Geometry: see drawing. Coordinates: mm, zero at the bounding-box minimum. Give positions to 0.01 mm unless a question says otherwise; leave off trailing zeros. Loops run counter-clockwise (first coordinate to the right, second up) from the corner with the lowest first, then second, coordinate; pieces in that order, holes last. Notation, with made-up numbers: (50.5, 48) - (82.5, 48) arc R13 ccw to (82.5, 70) - close; hole circle Ø3 at (70, 71.25). An arc over 180 degrees is marked (long way). Use one line per item in the form item = value.
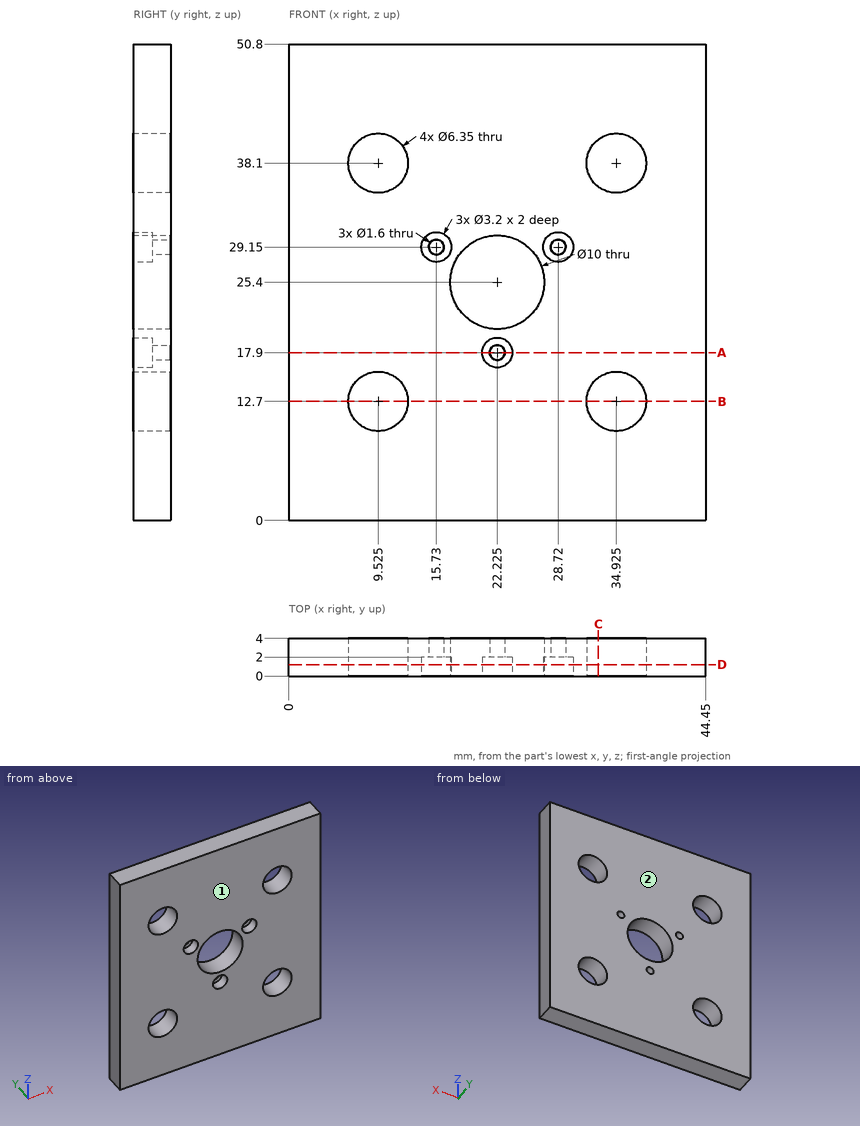
(1) Cut plane A-A (z = 17.9). Return the cut outline in (x, y) (3 decimals), plus the area to 3 significant figures.
Solution:
outline = (0, 0) - (20.625, 0) - (20.625, 2) - (21.425, 2) - (21.425, 4) - (0, 4) - close; (23.025, 2) - (23.825, 2) - (23.825, 0) - (44.45, 0) - (44.45, 4) - (23.025, 4) - close
area = 168 mm2
(2) Pull-direction query (Y, two-part tool) for the marked faces 1 and 2; classes: released by +Y, released by -Y, zero draft, split by the parting line, or undercut.
Solution:
face_1 = released by -Y
face_2 = released by +Y
(3) Material intervals for L1, parallel to X at y = 1.6, z = 38; L2, parallel to X at y = 0.85, z = 17.9 (3 decimals); L3, parallel to Z at x = 7.5, y = 3.1 (1 decimal), sorted ascending. Write a range as from..to.
Solution:
L1 = 0..6.35, 12.7..31.75, 38.1..44.45
L2 = 0..20.625, 23.825..44.45
L3 = 0..10.3, 15.1..35.7, 40.5..50.8
(4) Pin query (flat end, axial travel): P1, Ø1, axis at x = 28.5, z = 30, coming from the -Y side. Return the tip coordinate at first contact, or that it passes through.
Solution:
P1 = 2
(5) Cut plane D-D (y = 1.2). Give the number of separate pieces and of enclosed holes in the cut face, plus the area to 3 significant figures.
Solution:
separate_pieces = 1
enclosed_holes = 8
area = 2,030 mm2
(6) Cut plane B-B (z = 12.7). Return the cut outline in (x, y), plus the area to 3 significant figures.
Solution:
outline = (0, 0) - (6.35, 0) - (6.35, 4) - (0, 4) - close; (12.7, 0) - (31.75, 0) - (31.75, 4) - (12.7, 4) - close; (38.1, 0) - (44.45, 0) - (44.45, 4) - (38.1, 4) - close
area = 127 mm2
(7) Cut plane C-C (x = 33). Return the cut outline in (y, z) (1 decimal), plus the area to 3 significant figures.
Solution:
outline = (0, 0) - (4, 0) - (4, 10.2) - (0, 10.2) - close; (0, 15.2) - (4, 15.2) - (4, 35.6) - (0, 35.6) - close; (0, 40.6) - (4, 40.6) - (4, 50.8) - (0, 50.8) - close
area = 163 mm2
